Job drawing, mm, ordinate dimensions from the low corner. One solid piece. A direction names the side the tool comes from. Round coordinates to 2 decimals unless told otherwise and drop trailing zeros. Loops run counter-clockwise (first coordinate to the right, second up) from the corner with the lowest first, then second, coordinate; pieces in that order, holes last. Notation, with made-up numbers: M 19.25,-35 L 50.25,-35 A14 cw 50.25,-24 Z; hole C 18,5 d8. An arc over 180 degrees is marked long. Use one line per item in the form item = value. Start each with the question number.
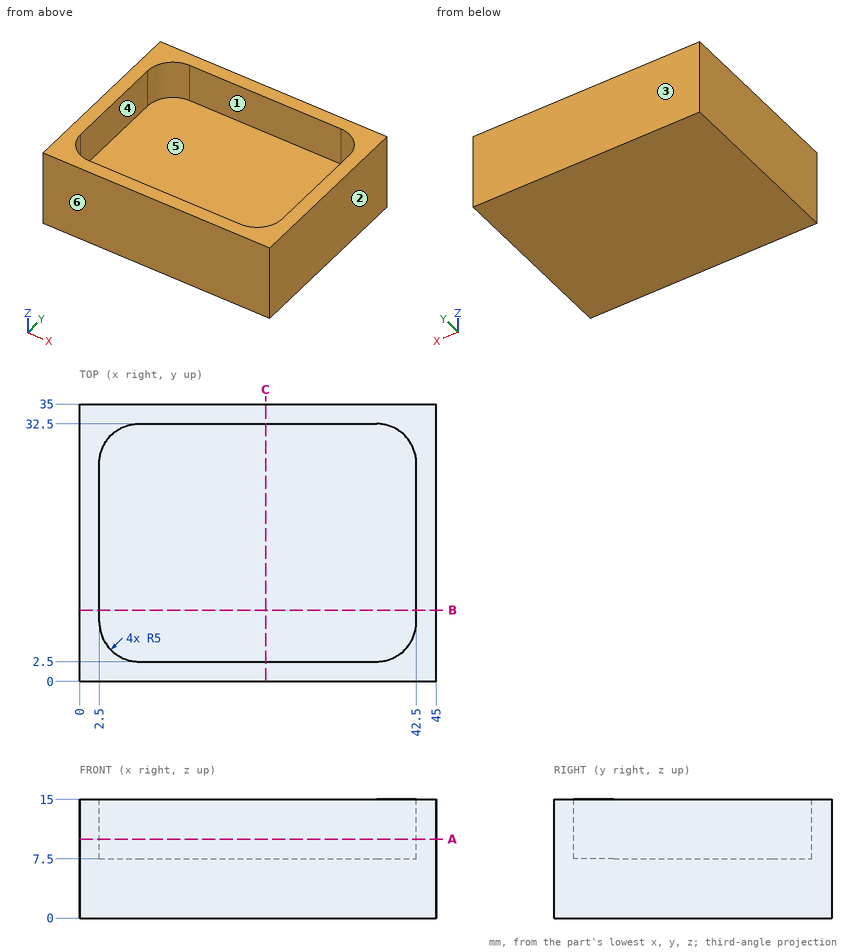
Q1. Wall check: probe 1 along X at (y, z) = (27.5, 13); probe 2 along Y at (x, z) = (27.5, 9.5); probe 3 along Z at (x, y) = (36.5, 12). Give the ranges that are in metal, low to high.
Q2. Saw through at A-A (z = 10). Give the cut face in (x, y).
Q3. Pull direction X, two halves, no side cores. Call the marked faces 1, 2, 3 and 4: pulls with the +X half, pulls with the -X half, needs draft (parallel to the pull), parting line crosses it, or undercut.
Q4. Drop a flat-ended pin along its axis: P1, Ø8, axis at x = 33.5, y = 8.5, coming from the +Z side. Give the stop position or say it passes through.
Q5. Saw through at B-B (y = 9). Give the cut face in (x, z).
Q6. Tool access for the marked faces 5 and 6: list every direction of +Z, -Z, +X, -X, +Y, -Y with a clear straight run to the whole face (end or side of a thin tool).
Q7. Saw through at C-C (x = 23.5). Give the cut face in (y, z).
Filled in:
q1.probe_1 = 0 to 2.5, 42.5 to 45
q1.probe_2 = 0 to 2.5, 32.5 to 35
q1.probe_3 = 0 to 7.5
q2.outline = M 0,0 L 45,0 L 45,35 L 0,35 Z; hole M 2.5,7.5 A5 ccw 7.5,2.5 L 37.5,2.5 A5 ccw 42.5,7.5 L 42.5,27.5 A5 ccw 37.5,32.5 L 7.5,32.5 A5 ccw 2.5,27.5 Z
q3.face_1 = undercut
q3.face_2 = pulls with the +X half
q3.face_3 = needs draft
q3.face_4 = undercut
q4.P1 = 7.5
q5.outline = M 0,0 L 45,0 L 45,15 L 42.5,15 L 42.5,7.5 L 2.5,7.5 L 2.5,15 L 0,15 Z
q6.face_5 = +Z
q6.face_6 = +Z, -Z, +X, -X, -Y
q7.outline = M 0,0 L 35,0 L 35,15 L 32.5,15 L 32.5,7.5 L 2.5,7.5 L 2.5,15 L 0,15 Z
